from build123d import *

# Parameters (mm, degrees)
SKETCH1_R                    = 17.9
BOSS_EXTRUDE1_DEPTH          = 50
SKETCH2_R                    = 6.5
BOSS_EXTRUDE2_DEPTH          = 4
SKETCH4_R                    = 5
BOSS_EXTRUDE3_DEPTH          = 3
BOSS_EXTRUDE4_DEPTH          = 11
BOSS_EXTRUDE4_DEPTH_BACK     = 59
SKETCH3_R                    = 1.6
SKETCH5_R                    = 17.9
SKETCH5_R_2                  = 17.5
BOSS_EXTRUDE5_DEPTH          = 1
SKETCH6_W                    = 0.5
SKETCH6_H                    = 3.8
BOSS_EXTRUDE6_DEPTH          = 7.5
SKETCH7_R                    = 1.25
CUT_EXTRUDE1_DEPTH           = 0.5
FILLET1_R                    = 1
FILLET1_OF_MIRROR3_R         = 1
FILLET2_R                    = 1
FILLET3_R                    = 1
M2_5X0_45_TAPPED_HOLE1_D     = 2.05
M2_5X0_45_TAPPED_HOLE1_DEPTH = 6.35
M2_5X0_45_TAPPED_HOLE1_TIP   = 0.615882135


with BuildPart() as part:
    # Sketch1 → Boss-Extrude1 (new body)
    with BuildSketch(Plane.XY):
        Circle(SKETCH1_R)
    extrude(amount=BOSS_EXTRUDE1_DEPTH)

    # Sketch2 → Boss-Extrude2 (add)
    with BuildSketch(Plane(origin=(0, 0, 0), x_dir=(-1, 0, 0), z_dir=(0, 0, -1))):
        Circle(SKETCH2_R)
    extrude(amount=BOSS_EXTRUDE2_DEPTH)

    # Sketch4 → Boss-Extrude3 (add)
    with BuildSketch(Plane.XY.offset(50)):
        Circle(SKETCH4_R)
    extrude(amount=BOSS_EXTRUDE3_DEPTH)

    # Sketch3 → Boss-Extrude4 (add, two sides: drawn at the far end of the back side and taken through both)
    with BuildSketch(Plane(origin=(0, 0, -4), x_dir=(-1, 0, 0), z_dir=(0, 0, -1)).offset(-BOSS_EXTRUDE4_DEPTH_BACK)):
        with Locations(Location((0, 0, 0), (0, 0, 180))):
            Circle(SKETCH3_R)
    extrude(amount=BOSS_EXTRUDE4_DEPTH + BOSS_EXTRUDE4_DEPTH_BACK)

    # Sketch5 → Boss-Extrude5 (add)
    with BuildSketch(Plane.XY.offset(50)):
        Circle(SKETCH5_R)
        Circle(SKETCH5_R_2, mode=Mode.SUBTRACT)
    extrude(amount=BOSS_EXTRUDE5_DEPTH)

    # Sketch6 → Boss-Extrude6 (add)
    with BuildSketch(Plane.XY.offset(50)):
        with Locations((-14.25, 0)):
            Rectangle(SKETCH6_W, SKETCH6_H)
    boss_extrude6 = extrude(amount=BOSS_EXTRUDE6_DEPTH)

    # Sketch7 → Cut-Extrude1 (cut)
    with BuildSketch(Plane.ZY.offset(14.5)):
        with Locations((55.6, 0)):
            Circle(SKETCH7_R)
    cut_extrude1 = extrude(amount=-CUT_EXTRUDE1_DEPTH, mode=Mode.SUBTRACT)

    # Fillet1
    fillet1_edges = [part.edges().sort_by_distance(p)[0] for p in [
        (-14.25, 1.9, 57.5),
        (-14.25, -1.9, 57.5),
    ]]
    fillet(fillet1_edges, radius=FILLET1_R)

    # Mirror3: Boss-Extrude6, Cut-Extrude1 across plane
    add(boss_extrude6.mirror(Plane(origin=(0, 0, 0), x_dir=(0, 0, 1), z_dir=(1, 0, 0))))
    add(cut_extrude1.mirror(Plane(origin=(0, 0, 0), x_dir=(0, 0, 1), z_dir=(1, 0, 0))), mode=Mode.SUBTRACT)

    # Fillet1 of Mirror3
    fillet1_of_mirror3_edges = [part.edges().sort_by_distance(p)[0] for p in [
        (14.25, 1.9, 57.5),
        (14.25, -1.9, 57.5),
    ]]
    fillet(fillet1_of_mirror3_edges, radius=FILLET1_OF_MIRROR3_R)

    # Fillet2
    fillet2_edges = [part.edges().sort_by_distance(p)[0] for p in [
        (-17.9, 0, 0),
    ]]
    fillet(fillet2_edges, radius=FILLET2_R)

    # Fillet3
    fillet3_edges = [part.edges().sort_by_distance(p)[0] for p in [
        (6.5, 0, -4),
    ]]
    fillet(fillet3_edges, radius=FILLET3_R)

    # M2.5x0.45 Tapped Hole1
    with Locations(Plane(origin=(0, 0, 0), x_dir=(-1, 0, 0), z_dir=(0, 0, -1))):
        with Locations((-12.5, 0), (12.5, 0)):
            Hole(M2_5X0_45_TAPPED_HOLE1_D / 2, depth=M2_5X0_45_TAPPED_HOLE1_DEPTH)
            with Locations((0, 0, -(M2_5X0_45_TAPPED_HOLE1_DEPTH + M2_5X0_45_TAPPED_HOLE1_TIP / 2))):  # 118° drill point
                Cone(0, M2_5X0_45_TAPPED_HOLE1_D / 2, M2_5X0_45_TAPPED_HOLE1_TIP, mode=Mode.SUBTRACT)


solid = part.part
The listing builds one solid part. Answer for the finished solid, in the listing's coordinates (mm). A direction names the side the tool comes from. Give positions to 0.01 mm unless a question says otherwise; leave off trailing zeros. Loops run counter-clockwise (first coordinate to the right, second up) from the corner with the lowest first, then second, coordinate; pieces in that order, holes last. Notation, with made-up numbers: M 31,62.5 L 71,62.5 A21 cw 71,78.5 Z; hole C 84.5,-12.75 d4. An arc over 180 degrees is marked long. Answer as CSV lines item,"result".
Item 1: Straight lines are drawn through the part: line 1 along Y through (x, z) = (0, 50.65); line 2 along X through (y, z) = (1, 54); line 3 along Y through (x, z) = (-14.4, 55.6). For each, find the intervals that lie inside material, in ascending order. Write a range as [from, to].
Values follow:
line 1,"y = [-17.9, -17.5], [-5, 5], [17.5, 17.9]"
line 2,"x = [-14.5, -14], [-1.25, 1.25], [14, 14.5]"
line 3,"y = [-1.9, -1.25], [1.25, 1.9]"
Item 2: The part is cut by section C-C (z = -10). Give the vertices of the cut face in (x, y).
Values follow:
outline,"C 0,0 d3.2"
Item 3: Which of the six approach directions +Z, -Z, +X, -X, +Y, -Y give full straight-line access (tool end or side, diameter ignored) to faces 4 (the cylindrical face through (-14.25, 0.38, 56.79)), 5 (the cylindrical face through (-14.2, -10.9, 25.6)), 6 (the flat face through (-14.5, 0, 54)), 7 (the cylindrical face through (-13.524, 0.045, 3.219)), 8 (the flat face through (0, 0, 55))?
Values follow:
face 4,"-X"
face 5,"+Z, -Z"
face 6,"+Z"
face 7,"-Z"
face 8,"+Z, +Y, -Y"
Item 4: Given pin 1 Ø6 at (x, y) = (4, -2.5) entering from -Z; pin 2 Ø11 at (x, y) = (1.5, 1) entering from +Z; pin 3 Ø1.5 at (y, z) = (12.5, 41.5) entering from +X, each flat-ended and moving along its own axis, determine where each tip first touches the part or whether it passes through.
Values follow:
pin 1,"stops at z = -4"
pin 2,"stops at z = 55"
pin 3,"stops at x = 13.5"
Item 5: The part is cut by section B-B (z = 26). Give the vertices of the cut face in (x, y), and give its area (3 significant figures).
Values follow:
outline,"C 0,0 d35.8"
area,"1,010 mm^2"
Item 6: The mould has two halves that part along Y. Classify faces 1 (the flat face through (1.3, 1.3, -4)), 2 (the cylindrical face through (1.526, -0.481, -9.423)), 3 (the cylindrical face through (11.476, 0.045, 3.219)): released by +Y, released by -Y, zero draft, split by the parting line, or undercut.
Values follow:
face 1,"zero draft"
face 2,"split by the parting line"
face 3,"undercut"
Item 7: The part is cut by section A-A (x = 0). Give the vertices of the cut face in (y, z), and give its area (3 significant figures).
Values follow:
outline,"M -17.9,1 A1 ccw -16.9,0 L -6.5,0 L -6.5,-3 A1 ccw -5.5,-4 L -1.6,-4 L -1.6,-15 L 1.6,-15 L 1.6,-4 L 5.5,-4 A1 ccw 6.5,-3 L 6.5,0 L 16.9,0 A1 ccw 17.9,1 L 17.9,51 L 17.5,51 L 17.5,50 L 5,50 L 5,53 L 1.6,53 L 1.6,55 L -1.6,55 L -1.6,53 L -5,53 L -5,50 L -17.5,50 L -17.5,51 L -17.9,51 Z"
area,"1,910 mm^2"
